from build123d import *

# Parameters (mm, degrees)
SKETCH1_R                                    = 60.625
SKETCH1_R_2                                  = 45
BOSS_EXTRUDE1_DEPTH                          = 4
SKETCH2_R                                    = 49
SKETCH2_R_2                                  = 45
BOSS_EXTRUDE2_DEPTH                          = 52
SKETCH4_W                                    = 13.25
SKETCH4_H                                    = 8
SKETCH4_W_2                                  = 8
SKETCH4_H_2                                  = 38
BOSS_EXTRUDE4_DEPTH                          = 13
BOSS_EXTRUDE5_DEPTH                          = 4
BOSS_EXTRUDE6_REACH                          = 104.405
SKETCH18_R                                   = 45.113728165
SKETCH18_R_2                                 = 38.5
SKETCH7_R                                    = 1.3
CUT_EXTRUDE4_DEPTH                           = 7.2
SKETCH9_W                                    = 10
SKETCH9_H                                    = 24
CUT_EXTRUDE7_DEPTH                           = 8
SKETCH11_R                                   = 7.5
CUT_EXTRUDE8_DEPTH                           = 20
CUT_EXTRUDE9_DEPTH                           = 101.273532203
CSK_FOR_M3_COUNTERSUNK_FLAT_HEAD_SCR_2_COUNT = 2
CSK_FOR_M3_COUNTERSUNK_FLAT_HEAD_SCR_2_PITCH = 77.781745931
CSK_FOR_M3_COUNTERSUNK_FLAT_HEAD_SCR_3_COUNT = 2
CSK_FOR_M3_COUNTERSUNK_FLAT_HEAD_SCR_3_PITCH = 110
CSK_FOR_M3_COUNTERSUNK_FLAT_HEAD_SCR_4_COUNT = 2
CSK_FOR_M3_COUNTERSUNK_FLAT_HEAD_SCR_4_PITCH = 77.781745931
SKETCH20_R                                   = 38.708370422
BOSS_EXTRUDE7_DEPTH                          = 5
SKETCH21_R                                   = 47
SKETCH21_R_2                                 = 40.5
CUT_EXTRUDE10_DEPTH                          = 2


with BuildPart() as part:
    # Sketch1 → Boss-Extrude1 (new body)
    with BuildSketch(Plane(origin=(0, 0, 0), x_dir=(1, 0, 0), z_dir=(0, 1, 0))):
        with Locations(Location((0, 0, 0), (0, 0, 270))):
            Circle(SKETCH1_R)
        with Locations(Location((0, 0, 0), (0, 0, 270))):
            Circle(SKETCH1_R_2, mode=Mode.SUBTRACT)
    extrude(amount=BOSS_EXTRUDE1_DEPTH)

    # Sketch2 → Boss-Extrude2 (add)
    with BuildSketch(Plane(origin=(0, 4, 0), x_dir=(1, 0, 0), z_dir=(0, 1, 0))):
        with Locations(Location((0, 0, 0), (0, 0, 90))):
            Circle(SKETCH2_R)
        with Locations(Location((0, 0, 0), (0, 0, 270))):
            Circle(SKETCH2_R_2, mode=Mode.SUBTRACT)
    extrude(amount=BOSS_EXTRUDE2_DEPTH)

    # Sketch4 → Boss-Extrude4 (add, symmetric)
    with BuildSketch(Plane.XY):
        with Locations((-38.375, 34)):
            Rectangle(SKETCH4_W, SKETCH4_H)
        Polygon((-31.75, 30), (-45, 30), (-45, 16.75), align=None)
        with Locations((15.25, 19)):
            Rectangle(SKETCH4_W_2, SKETCH4_H_2)
    extrude(amount=BOSS_EXTRUDE4_DEPTH, both=True)


with BuildPart() as boss_extrude4_piece_1:
    # of the separate pieces the step leaves, piece 1, a body of its own (boss_extrude4_pieces)
    add(part.part.solids().sort_by_distance((0, 0, 60.625))[0])



with BuildPart() as boss_extrude4_piece_2:
    # of the separate pieces the step leaves, piece 2, a body of its own (boss_extrude4_pieces)
    add(part.part.solids().sort_by_distance((11.25, 38, -13))[0])


with BuildPart() as boss_extrude4_piece_1_1:
    add(boss_extrude4_piece_1.part)

    add(boss_extrude4_piece_2.part)  # Boss-Extrude5 merges Boss-Extrude4 piece 2
    # Sketch5 → Boss-Extrude5 (add)
    with BuildSketch(Plane.XZ):
        with BuildLine():
            Line((11.25, 13), (29.067400866, 34.352382842))
            ThreePointArc((29.067400866, 34.352382842), (45, 0), (29.067400866, -34.352382842))
            Line((29.067400866, -34.352382842), (11.25, -13))
            Line((11.25, -13), (11.25, 13))
        make_face()
    extrude(amount=-BOSS_EXTRUDE5_DEPTH)

    # Boss-Extrude6: up to this face of the body (flat: up to its plane)
    boss_extrude6_end = Plane(boss_extrude4_piece_1_1.part.faces().sort_by_distance((12.964733944, 0, 0))[0])
    # Sketch18 → Boss-Extrude6 (add, up to the picked face)
    with BuildSketch(Plane(origin=(0, 56, 0), x_dir=(1, 0, 0), z_dir=(0, 1, 0)), mode=Mode.PRIVATE) as boss_extrude6_sk1:
        Circle(SKETCH18_R)
        with Locations(Location((0, 0, 0), (0, 0, 270))):
            Circle(SKETCH18_R_2, mode=Mode.SUBTRACT)
    boss_extrude6_tool1 = split(extrude(boss_extrude6_sk1.sketch, amount=-BOSS_EXTRUDE6_REACH, mode=Mode.PRIVATE), bisect_by=boss_extrude6_end, keep=Keep.BOTH, mode=Mode.PRIVATE)
    add(boss_extrude6_tool1.solids().sort_by(Axis((-43.837719, 56, 0), (0, -1, 0)))[0])

    # Sketch7 → Cut-Extrude4 (cut)
    with BuildSketch(Plane(origin=(0, 38, 0), x_dir=(1, 0, 0), z_dir=(0, 1, 0))):
        with Locations(Location((-34.25, 5, 0), (0, 0, 180))):
            Circle(SKETCH7_R)
        with Locations(Location((-34.25, -5, 0), (0, 0, 180))):
            Circle(SKETCH7_R)
        with Locations(Location((13.75, 5, 0), (0, 0, 180))):
            Circle(SKETCH7_R)
        with Locations(Location((13.75, -5, 0), (0, 0, 180))):
            Circle(SKETCH7_R)
    extrude(amount=-CUT_EXTRUDE4_DEPTH, mode=Mode.SUBTRACT)

    # Sketch9 → Cut-Extrude7 (cut)
    with BuildSketch(Plane.ZY.offset(-11.25)):
        with Locations((0, 17)):
            Rectangle(SKETCH9_W, SKETCH9_H)
    extrude(amount=-CUT_EXTRUDE7_DEPTH, mode=Mode.SUBTRACT)

    # Sketch11 → Cut-Extrude8 (cut)
    with BuildSketch(Plane(origin=(49, 0, 0), x_dir=(0, 0, -1), z_dir=(1, 0, 0))):
        with Locations((0, 14)):
            Circle(SKETCH11_R)
    extrude(amount=-CUT_EXTRUDE8_DEPTH, mode=Mode.SUBTRACT)

    # Sketch12 → Cut-Extrude9 (cut, through all)
    # profile 1 of 2: a face of its own
    with BuildSketch(Plane(origin=(0, 4, 0), x_dir=(1, 0, 0), z_dir=(0, 1, 0))):
        with BuildLine():
            Line((19.25, -13), (11.25, -13))
            Line((11.25, -13), (24.902812686, -29.361538112))
            ThreePointArc((24.902812686, -29.361538112), (38.5, 0), (24.902812686, 29.361538112))
            Line((24.902812686, 29.361538112), (11.25, 13))
            Line((11.25, 13), (19.25, 13))
            Line((19.25, 13), (19.25, -13))
        make_face()
        with BuildLine():
            Line((27.25, -13.699908759), (27.25, 13.699908759))
            ThreePointArc((27.25, 13.699908759), (30.5, 0), (27.25, -13.699908759))
        make_face(mode=Mode.SUBTRACT)
    # profile 2 of 2: a face of its own
    with BuildSketch(Plane(origin=(0, 4, 0), x_dir=(1, 0, 0), z_dir=(0, 1, 0))):
        with BuildLine():
            ThreePointArc((27.25, -13.699908759), (30.5, 0), (27.25, 13.699908759))
            Line((27.25, 13.699908759), (27.25, -13.699908759))
        make_face()
    extrude(amount=-CUT_EXTRUDE9_DEPTH, mode=Mode.SUBTRACT)


with BuildPart() as cut_extrude9_piece_1:
    # of the separate pieces the step leaves, piece 1, a body of its own (cut_extrude9_pieces)
    add(boss_extrude4_piece_1_1.part.solids().sort_by_distance((0, 0, 38.5))[0])

    # Sketch17 → CSK for M3 Countersunk Flat Head Screw1 (revolve, cut)
    with BuildSketch(Plane(origin=(-38.890872965, 4, -38.890872965), x_dir=(0, 0, 1), z_dir=(1, 0, 0))):
        Polygon((0, 0), (0, 4), (1.7, 4), (1.7, 1.45), (3.15, 0), align=None)
    csk_for_m3_countersunk_flat_head_screw1 = revolve(axis=Axis((-38.890872965, 10.35, -38.890872965), (0, -1, 0)), mode=Mode.SUBTRACT)

    # CSK for M3 Countersunk Flat Head Scr 2: CSK for M3 Countersunk Flat Head Screw1 ×2
    with Locations(*[(0, 0, i * CSK_FOR_M3_COUNTERSUNK_FLAT_HEAD_SCR_2_PITCH) for i in range(1, CSK_FOR_M3_COUNTERSUNK_FLAT_HEAD_SCR_2_COUNT)]):
        add(csk_for_m3_countersunk_flat_head_screw1, mode=Mode.SUBTRACT)

    # CSK for M3 Countersunk Flat Head Scr 3: CSK for M3 Countersunk Flat Head Screw1 ×2
    with Locations(*[Vector(0.7071067811865713, 0, 0.7071067811865237) * (i * CSK_FOR_M3_COUNTERSUNK_FLAT_HEAD_SCR_3_PITCH) for i in range(1, CSK_FOR_M3_COUNTERSUNK_FLAT_HEAD_SCR_3_COUNT)]):
        add(csk_for_m3_countersunk_flat_head_screw1, mode=Mode.SUBTRACT)

    # CSK for M3 Countersunk Flat Head Scr 4: CSK for M3 Countersunk Flat Head Screw1 ×2
    with Locations(*[(i * CSK_FOR_M3_COUNTERSUNK_FLAT_HEAD_SCR_4_PITCH, 0, 0) for i in range(1, CSK_FOR_M3_COUNTERSUNK_FLAT_HEAD_SCR_4_COUNT)]):
        add(csk_for_m3_countersunk_flat_head_screw1, mode=Mode.SUBTRACT)



with BuildPart() as cut_extrude9_piece_2:
    # of the separate pieces the step leaves, piece 2, a body of its own (cut_extrude9_pieces)
    add(boss_extrude4_piece_1_1.part.solids().sort_by_distance((11.25, 38, -13))[0])


with BuildPart() as cut_extrude9_piece_1_1:
    add(cut_extrude9_piece_1.part)

    add(cut_extrude9_piece_2.part)  # Boss-Extrude7 merges Cut-Extrude9 piece 2
    # Sketch20 → Boss-Extrude7 (add)
    with BuildSketch(Plane(origin=(0, 5, 0), x_dir=(1, 0, 0), z_dir=(0, 1, 0))):
        Circle(SKETCH20_R)
    extrude(amount=-BOSS_EXTRUDE7_DEPTH)

    # Sketch21 → Cut-Extrude10 (cut)
    with BuildSketch(Plane(origin=(0, 56, 0), x_dir=(1, 0, 0), z_dir=(0, 1, 0))):
        with Locations(Location((0, 0, 0), (0, 0, 270))):
            Circle(SKETCH21_R)
        with Locations(Location((0, 0, 0), (0, 0, 270))):
            Circle(SKETCH21_R_2, mode=Mode.SUBTRACT)
    extrude(amount=-CUT_EXTRUDE10_DEPTH, mode=Mode.SUBTRACT)


solid = cut_extrude9_piece_1_1.part
Geometry: final body of the model. Coordinates: model frame, mm. A direction names the side the tool comes from. Round coordinates to 2 decimals unless told otherwise and drop trailing zeros. Loops run counter-clockwise (first coordinate to the right, second up) from the corner with the lowest first, then second, coordinate; pieces in that order, holes last. Notation, with made-up numbers: (28.25, 81.5) - (47.25, 81.5) arc R26 ccw to (47.25, 100.5) - close; hole circle Ø10 at (51.5, 55). An arc over 180 degrees is marked (long way). Write each question's results on one line, items separated by ' | '. Start each with the question number.
1) Line query: probe 1 along Z at (x, y) = (-34, 36); probe 2 along X at (y, z) = (11, -9.5); probe 3 along Z at (x, y) = (13, 34). Output: solid intervals per line, ascending. Write a range as [from, to].
2) Cut plane D-D on x = 0. Return loops of the section in (y, z) (3 decimals).
3) Cut plane C-C on y = 15.5. Return loops of the section in (x, z), then the cut area to 3 significant figures.
4) Cut plane B-B on z = 0. Count the separate pieces of the cut face and the enclosed holes in it, then the cut area to 3 significant figures.
5) Mould query, pull axis X, two halves, no side actions, for faces 1 (the face through (15, 38, 0)), 2 (the face through (40, 56, 25)), 3 (the face through (38.82, 1.29, -40.59)), 4 (the face through (-14.718, 29.636, -46.737)). Classes: released by +X, released by -X, zero draft, split by the parting line, or undercut.
6) Cut plane A-A on y = 27. Return loops of the section in (x, z), then the cut area to 3 significant figures.
7) Access query for faces 5 (the face through (43.46, 11.13, -6.93)), 6 (the face through (15, 17, -5)), 7 (the face through (15, 22, -13)). Directions: +Z, -Z, +X, -X, +Y, -Y. A direction counts if a zero-diameter tool reaches every point of the face in a straight line with its end or side. Return the directions, or none.
8) First-contact query: P1, Ø5, axis at y = 46.5, z = -23.5, coming from the -X side; P2, Ø6, axis at y = 19.5, z = -3.5, coming from the +X side; P3, Ø4.5, axis at x = -38.89, z = 38.89, coming from the +Y side; P4, Ø4, axis at x = -38.5, z = 21, coming from the -Y side. Flat tips, straight axial feed; report the tip coordinate or a pass-through.
Verdict:
1) probe 1: z = [-35.28, -18.06], [-13, -6.28], [-3.72, 3.72], [6.28, 13], [18.06, 35.28] | probe 2: x = [-48.07, -37.31], [11.25, 19.25], [37.31, 48.07] | probe 3: z = [-47.24, -36.24], [-13, -6.06], [-3.94, 3.94], [6.06, 13], [36.24, 47.24]
2) outline: (0, -60.625) - (4, -60.625) - (4, -49) - (56, -49) - (56, -47) - (54, -47) - (54, -40.5) - (56, -40.5) - (56, -38.5) - (5, -38.5) - (5, 38.5) - (56, 38.5) - (56, 40.5) - (54, 40.5) - (54, 47) - (56, 47) - (56, 49) - (4, 49) - (4, 60.625) - (0, 60.625) - close
3) outline: (11.25, -13) - (19.25, -13) - (19.25, -5) - (11.25, -5) - close; (11.25, 5) - (19.25, 5) - (19.25, 13) - (11.25, 13) - close; (37.79, -7.35) arc R38.5 cw (long way) to (37.79, 7.35) - (48.45, 7.35) arc R49 ccw (long way) to (48.45, -7.35) - close | area: 2,860 mm2
4) separate pieces: 3 | enclosed holes: 0 | area: 1,620 mm2
5) face 1: undercut | face 2: zero draft | face 3: undercut | face 4: split by the parting line
6) outline: circle Ø98 at (0, 0); (11.25, -13) - (19.25, -13) - (19.25, -5) - (11.25, -5) - close; (11.25, 5) - (19.25, 5) - (19.25, 13) - (11.25, 13) - close; hole (-36.24, -13) arc R38.5 ccw (long way) to (-36.24, 13) - (-34.75, 13) - (-34.75, -13) - close | area: 3,090 mm2
7) face 5: +X | face 6: none | face 7: +Y
8) P1: stops at x = -44.27 | P2: stops at x = 48.99 | P3: stops at y = 3.1 | P4: stops at y = 0
